Read the model definition and answer for the solid it produces. Units are mm, in the model's axes. A direction names the side the tool comes from. Give positions to 0.01 mm unless a question says otherwise; leave off trailing zeros. Write each loop counter-clockwise with the first axis right and the second up, starting at its lowest first coordinate (ties: lowest second). Pieces come first, ordered by that corner, then holes.
```python
from build123d import *

# Parameters (mm, degrees)
F0_W     = 55
F0_H     = 55
F1_DEPTH = 1.6
F2_W     = 3
F2_H     = 6.9
F3_DEPTH = 8
F4_R     = 2.5
F5_DEPTH = 54.801


with BuildPart() as f1:
    # F0 (on Top) → F1 (new body)
    with BuildSketch(Plane.XY):
        Rectangle(F0_W, F0_H)
    extrude(amount=F1_DEPTH)

    # F2 (on face) → F3 (join)
    with BuildSketch(Plane.XY.offset(1.6)):
        with Locations((25.8, 24.05)):
            Rectangle(F2_W, F2_H)
        with Locations((25.8, -24.05)):
            Rectangle(F2_W, F2_H)
        with Locations((-25.8, -24.05)):
            Rectangle(F2_W, F2_H)
        with Locations((-25.8, 24.05)):
            Rectangle(F2_W, F2_H)
    extrude(amount=F3_DEPTH)

    # F4 (on face) → F5 (cut, through all)
    with BuildSketch(Plane.YZ.offset(27.3)):
        with Locations((24.05, 5.8)):
            Circle(F4_R)
        with Locations((-24.05, 5.8)):
            Circle(F4_R)
    extrude(amount=-F5_DEPTH, mode=Mode.SUBTRACT)


solid = f1.part
```
Item 1: Section B-B (y = 24.05) is taken. Write down the section's boundary in (x, z).
Result set:
outline: (-27.5, 0) - (27.5, 0) - (27.5, 1.6) - (27.3, 1.6) - (27.3, 3.3) - (24.3, 3.3) - (24.3, 1.6) - (-24.3, 1.6) - (-24.3, 3.3) - (-27.3, 3.3) - (-27.3, 1.6) - (-27.5, 1.6) - close; (-27.3, 8.3) - (-24.3, 8.3) - (-24.3, 9.6) - (-27.3, 9.6) - close; (24.3, 8.3) - (27.3, 8.3) - (27.3, 9.6) - (24.3, 9.6) - close
Item 2: Each of these flat-tipped pins is pushed along its axis until it touches: pin 1 Ø5.5 at (y, z) = (24.5, 7) entering from +X; pin 2 Ø2 at (y, z) = (23, 6.5) entering from -X; pin 3 Ø3.5 at (y, z) = (23, 4.5) entering from -X; pin 4 Ø2 at (x, y) = (-14.5, 2) entering from +Z. Where does it stop, or does it pass through?
Result set:
pin 1: stops at x = 27.3
pin 2: passes through
pin 3: stops at x = -27.3
pin 4: stops at z = 1.6
Item 3: Section C-C (x = 15.5) is taken. Write down the section's boundary in (y, z).
Result set:
outline: (-27.5, 0) - (27.5, 0) - (27.5, 1.6) - (-27.5, 1.6) - close
Item 4: Which of the six approach directions +Z, -Z, +X, -X, +Y, -Y give full straight-line access (tool end or side, diameter ignored) to faces 1 (the flat face through (-26, -20.6, 6)), 2 (the flat face through (27.3, -26, 4)), 3 (the flat face through (-24.3, -26, 4)), 4 (the flat face through (-27.3, 22, 4))?
Result set:
face 1: +Z, +X, -X
face 2: +Z, +X, +Y, -Y
face 3: +Z, +Y, -Y
face 4: +Z, -X, +Y, -Y
Item 5: Section A-A (z = 5.8) is taken. Give the number of separate pieces and of enclosed holes in the cut face, and give its area (3 significant figures).
Result set:
separate pieces: 8
enclosed holes: 0
area: 22.8 mm2
Item 6: Find the intervals of material crossed by line 1 along X through (y, z) = (21, 6); line 2 along Z through (x, y) = (25.1, 24.05); line 3 along Z through (x, y) = (17, -23.5), in increasing order.
Result set:
line 1: x = -27.3 to -24.3, 24.3 to 27.3
line 2: z = 0 to 3.3, 8.3 to 9.6
line 3: z = 0 to 1.6
Item 7: Determine the mould class of faces 5 (the flat face through (0, 0, 0)), 6 (the flat face through (26, -20.6, 6)), 7 (the cylindrical face through (25.82, 22.21, 7.49)) for opening direction Z: pulls with the +Z half, pulls with the -Z half, needs draft (parallel to the pull), parting line crosses it, or undercut.
Result set:
face 5: pulls with the -Z half
face 6: needs draft
face 7: undercut
